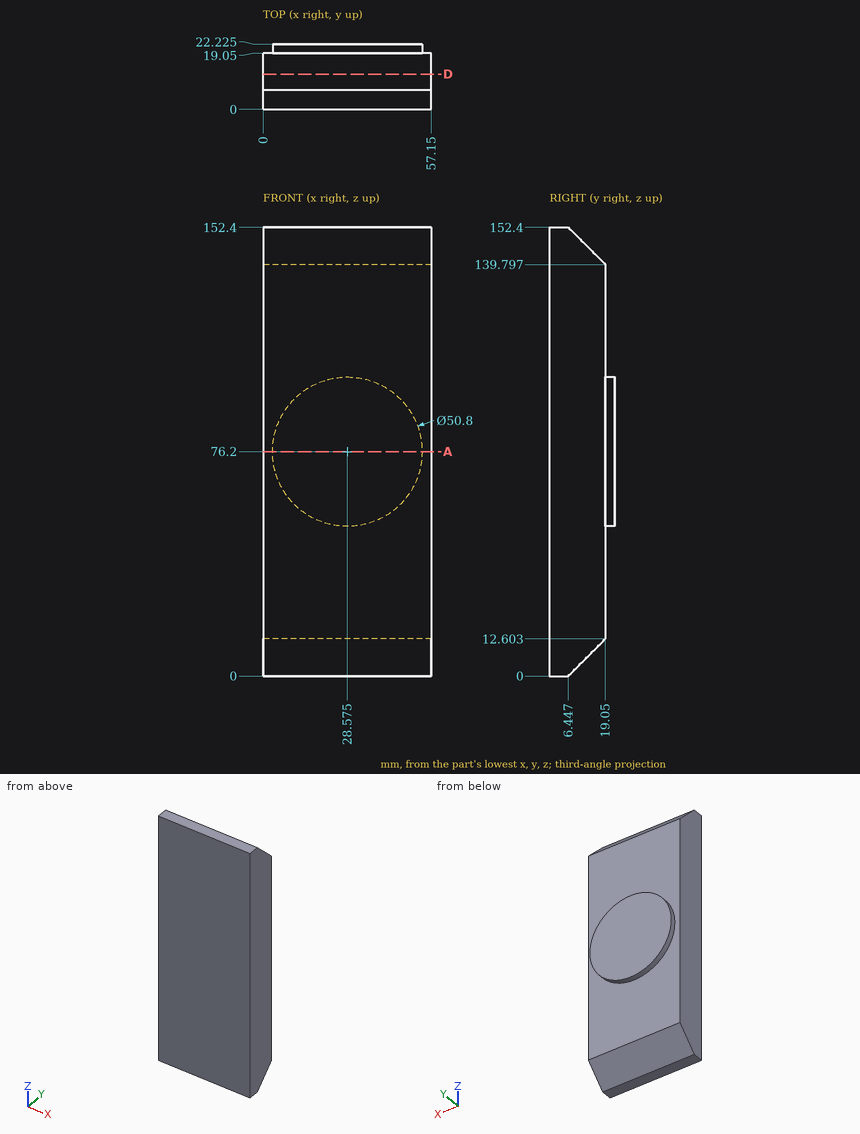
Here's the drawing with two shaded views (mm, measured from the low corner). I have some questions. Coordinates: 2 decimals unless noted, no trailing zeros. Order: outer loops, then holes, each group sorted by start corner. A loop starts at its lowest first (then second) coordinate and runs counter-clockwise, first axis right, second up. Notation, with made-up numbers: (73.25, -13.75) - (118.25, -13.75) arc R21 ccw to (118.25, 10.25) - close; hole circle Ø1 at (18.25, 81.25). An arc over 180 degrees is marked (long way). Use CSV: the item, a comma, the result in double quotes. Start each with the question number.
1. Suppose I cut it at D-D on y = 12. List the corners of the cut face in (x, z) for me, then the cut area to 4 significant figures.
2. Suppose I cut it at A-A on z = 76.2. List the corners of the cut face in (x, y) for me (3 decimals).
3. I'm going to push flat-ended pins straight in: pin 1 (5 mm diameter, centred on x = 50, z = 133.5, fed in from +Y); pin 2 (5 mm diameter, centred on x = 27.5, y = 16, fed in from -Z). Where does each tip first touch, or does it pass through?
4. Please list where these lines run through material, in increasing order: line 1 (Y direction, x = 12.5, z = 109); line 2 (Z direction, x = 16.5, y = 16); line 3 (Z direction, x = 4.5, y = 11.5). Write a range as from..to.
Output:
1,outline,"(0, 5.55) - (57.15, 5.55) - (57.15, 146.85) - (0, 146.85) - close"
1,area,"8,075 mm2"
2,outline,"(0, 0) - (57.15, 0) - (57.15, 19.05) - (53.975, 19.05) - (53.975, 22.225) - (3.175, 22.225) - (3.175, 19.05) - (0, 19.05) - close"
3,pin 1,"stops at y = 19.05"
3,pin 2,"stops at z = 7.05"
4,line 1,"y = 0..19.05"
4,line 2,"z = 9.55..142.85"
4,line 3,"z = 5.05..147.35"
